Check sheet for the modelled part. Datum: model origin and axes. Units: mm. Face numbers are marked on the shaded views. A direction names the side the tool comes from. Round coordinates to 2 decimals unless told otherwise and drop trailing zeros. Write each loop counter-clockwise with the first axis right and the second up, starting at its lowest first coordinate (ties: lowest second). Pieces come first, ordered by that corner, then holes. Notation, with made-up numbers: (40, 86.5) -> (48, 86.5) arc R14 ccw to (48, 106.5) -> close; hole circle Ø10 at (78, 70). An arc over 180 degrees is marked (long way). Put each result on its own line as item: value. Start each with the question number.
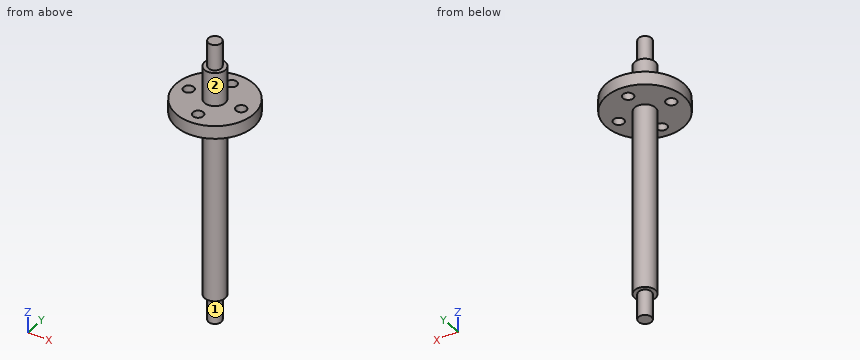
from build123d import *

# Parameters (mm, degrees)
SKETCH1_R           = 4
BOSS_EXTRUDE1_DEPTH = 109.95
SKETCH2_R           = 4
SKETCH2_R_2         = 2.5
CUT_EXTRUDE1_DEPTH  = 10
SKETCH3_R           = 15
SKETCH3_R_2         = 2
BOSS_EXTRUDE2_DEPTH = 5


with BuildPart() as part:
    # Sketch1 → Boss-Extrude1 (new body)
    with BuildSketch(Plane.XY):
        Circle(SKETCH1_R)
    extrude(amount=BOSS_EXTRUDE1_DEPTH)

    # Sketch2 → Cut-Extrude1 (cut)
    with BuildSketch(Plane(origin=(0, 0, 0), x_dir=(-1, 0, 0), z_dir=(0, 0, -1))):
        Circle(SKETCH2_R)
        Circle(SKETCH2_R_2, mode=Mode.SUBTRACT)
    cut_extrude1 = extrude(amount=-CUT_EXTRUDE1_DEPTH, mode=Mode.SUBTRACT)

    # Mirror1: Cut-Extrude1 across plane
    add(cut_extrude1.mirror(Plane.XY.offset(54.975)), mode=Mode.SUBTRACT)

    # Sketch3 → Boss-Extrude2 (add)
    with BuildSketch(Plane.XY.offset(81.95)):
        Circle(SKETCH3_R)
        with Locations((0, 10)):
            Circle(SKETCH3_R_2, mode=Mode.SUBTRACT)
        with Locations((10, 0)):
            Circle(SKETCH3_R_2, mode=Mode.SUBTRACT)
        with Locations((0, -10)):
            Circle(SKETCH3_R_2, mode=Mode.SUBTRACT)
        with Locations((-10, 0)):
            Circle(SKETCH3_R_2, mode=Mode.SUBTRACT)
    extrude(amount=BOSS_EXTRUDE2_DEPTH)


solid = part.part
1. Gauge pin test, flat ends, axial feed: P1, Ø12, axis at x = 11, y = -9.5, coming from the +Z side; P2, Ø5, axis at x = 10, y = 0, coming from the -Z side; P3, Ø1.5, axis at y = 4, z = 29.5, coming from the +X side. Record the tip position at first contact, or that the pin passes through.
2. Section check A-A, the plane x = 0. Enter the section's corners in (y, z), then the cut area to 3 significant figures.
3. Access from +Z, -Z, +X, -X, +Y, -Y to the whole of each face (thin tool, end or side, straight path). Record for the marked faces 1 and 2.
4. Section check C-C, the plane x = -11. Enter the section's corners in (y, z), then the cut area to 3 significant figures.
5. Material ranges on L1, parallel to Y at x = 0, z = 85.3; L2, parallel to Z at x = 8.5, y = 4; L3, parallel to X at y = -9, z = 82.5, recorded low to high. Write a range as [from, to].
6. Section check D-D, the plane y = -10. Enter the section's corners in (x, z), then the cut area to 3 significant figures.
Reply:
1. P1: stops at z = 86.95
1. P2: stops at z = 81.95
1. P3: stops at x = 2.33
2. outline: (-15, 81.95) -> (-12, 81.95) -> (-12, 86.95) -> (-15, 86.95) -> close; (-8, 81.95) -> (-4, 81.95) -> (-4, 10) -> (-2.5, 10) -> (-2.5, 0) -> (2.5, 0) -> (2.5, 10) -> (4, 10) -> (4, 81.95) -> (8, 81.95) -> (8, 86.95) -> (4, 86.95) -> (4, 99.95) -> (2.5, 99.95) -> (2.5, 109.95) -> (-2.5, 109.95) -> (-2.5, 99.95) -> (-4, 99.95) -> (-4, 86.95) -> (-8, 86.95) -> close; (12, 81.95) -> (15, 81.95) -> (15, 86.95) -> (12, 86.95) -> close
2. area: 890 mm2
3. face 1: -Z
3. face 2: +Z
4. outline: (-10.2, 81.95) -> (-1.73, 81.95) -> (-1.73, 86.95) -> (-10.2, 86.95) -> close; (1.73, 81.95) -> (10.2, 81.95) -> (10.2, 86.95) -> (1.73, 86.95) -> close
4. area: 84.7 mm2
5. L1: y = [-15, -12], [-8, 8], [12, 15]
5. L2: z = [81.95, 86.95]
5. L3: x = [-12, -1.73], [1.73, 12]
6. outline: (-11.18, 81.95) -> (-2, 81.95) -> (-2, 86.95) -> (-11.18, 86.95) -> close; (2, 81.95) -> (11.18, 81.95) -> (11.18, 86.95) -> (2, 86.95) -> close
6. area: 91.8 mm2
